CAD build for the part. Positions are in the model's coordinates, mm. Face numbers are marked on the shaded views. A direction names the side the tool comes from. Round coordinates to 2 decimals unless told otherwise and drop trailing zeros. Order: outer loops, then holes, each group sorted by start corner. A loop starts at its lowest first (then second) coordinate and runs counter-clockwise, first axis right, second up. Notation, with made-up numbers: M 65.5,-10 L 82.5,-10 A18 cw 82.5,-5 Z; hole C 52,19.25 d5. An arc over 180 degrees is marked long. Answer as CSV lines item,"result". Start each with the question number.
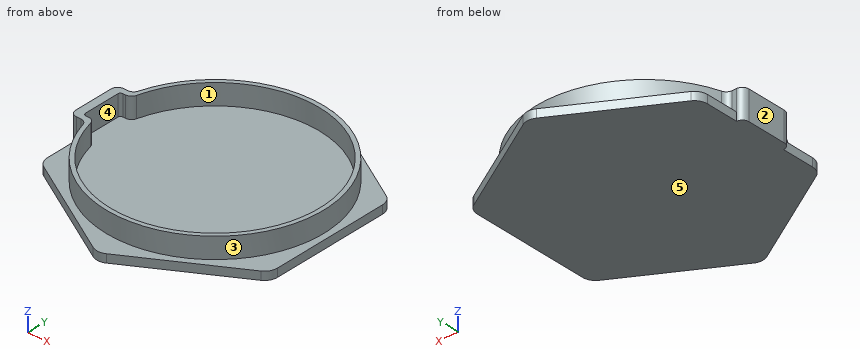
```python
from build123d import *

# Parameters (mm, degrees)
F1_DEPTH = 3.9878
F2_W     = 3.175
F2_H     = 25.4
F3_DEPTH = 3.9878
F5_DEPTH = 9.9822
F6_R     = 6.35
F7_R     = 1.27
F8_R     = 3.175


with BuildPart() as f1:
    # F0 (on Top) → F1 (new body)
    with BuildSketch(Plane.XY):
        Polygon((55.499, 32.042363), (0, 64.084725), (-55.499, 32.042363), (-55.499, -32.042363), (0, -64.084725), (55.499, -32.042363), align=None)
    extrude(amount=F1_DEPTH)

    # F2 (on face) → F3 (join, through all)
    with BuildSketch(Plane.XY.offset(3.9878)):
        with Locations((-57.0865, 0)):
            Rectangle(F2_W, F2_H)
    extrude(amount=-F3_DEPTH)

    # F4 (on face) → F5 (join)
    with BuildSketch(Plane.XY.offset(3.9878)):
        with BuildLine():
            Line((-55.499, -12.7), (-50.955694, -12.7))
            ThreePointArc((-50.955694, -12.7), (52.5145, 0), (-50.955694, 12.7))
            Line((-50.955694, 12.7), (-55.499, 12.7))
            Line((-55.499, 12.7), (-58.674, 12.7))
            Line((-58.674, 12.7), (-58.674, -12.7))
            Line((-58.674, -12.7), (-55.499, -12.7))
        make_face()
        with BuildLine():
            ThreePointArc((-49.483177, 9.9949), (50.4825, 0), (-49.483177, -9.9949))
            Line((-49.483177, -9.9949), (-54.690177, -9.9949))
            Line((-54.690177, -9.9949), (-54.690177, 9.9949))
            Line((-54.690177, 9.9949), (-49.483177, 9.9949))
        make_face(mode=Mode.SUBTRACT)
    extrude(amount=F5_DEPTH)

    # F6
    f6_edges = [f1.edges().sort_by_distance(p)[0] for p in [
        (-55.499, -32.042363, 1.9939),
        (0, -64.084725, 1.9939),
        (55.499, -32.042363, 1.9939),
        (55.499, 32.042363, 1.9939),
        (0, 64.084725, 1.9939),
        (-55.499, 32.042363, 1.9939),
    ]]
    fillet(f6_edges, radius=F6_R)

    # F7
    f7_edges = [f1.edges().sort_by_distance(p)[0] for p in [
        (-54.690177, -9.9949, 8.9789),
        (-54.690177, 9.9949, 8.9789),
    ]]
    fillet(f7_edges, radius=F7_R)

    # F8
    f8_edges = [f1.edges().sort_by_distance(p)[0] for p in [
        (-49.483177, -9.9949, 8.9789),
        (-49.483177, 9.9949, 8.9789),
        (-50.955694, 12.7, 8.9789),
        (-58.674, 12.7, 6.985),
        (-58.674, -12.7, 6.985),
        (-50.955694, -12.7, 8.9789),
    ]]
    fillet(f8_edges, radius=F8_R)


solid = f1.part
```
Q1. Band-saw the part on C-C, the plane y = -47.5. Write the cut outline in (x, z).
Q2. Drop flat-ended pins along their axis: P1, Ø2.5, axis at x = -54.5, z = 7.5, coming from the +Y side; P2, Ø6, axis at x = 31, z = 1.5, coming from the -Y side; P3, Ø2, axis at x = -25.5, y = -31, coming from the +Z side. Give the stop position or say it passes through.
Q3. Mould opens along X. For the marked faces 3, 4 and 5 say: +X half, -X half, draft (parallel to the pull), parting line (faces both ways), or undercut.
Q4. Band-saw the part on B-B, the plane y = 0. Write the cut outline in (x, z).
Q5. Tool access for the marked faces 1 and 2: list every direction of +Z, -Z, +X, -X, +Y, -Y with a clear straight run to the whole face (end or side of a thin tool).
Q6. Band-saw the part on A-A, the plane x = 0. Write the cut outline in (y, z).
Q7. Probe line 1 along X through (y, z) = (0, 8); line 2 along Y through (x, z) = (0, 10.5); line 3 along Z through (x, y) = (-44, 16.5). List the from-to ranges inside material, lowest first. Write a range as from..to.
Answer:
1,outline,"M -28.73,0 L 28.73,0 L 28.73,3.99 L 22.39,3.99 L 22.39,13.97 L 17.09,13.97 L 17.09,3.99 L -17.09,3.99 L -17.09,13.97 L -22.39,13.97 L -22.39,3.99 L -28.73,3.99 Z"
2,P1,"stops at y = 12.7"
2,P2,"stops at y = -47.92"
2,P3,"stops at z = 3.99"
3,face 3,"parting line"
3,face 4,"undercut"
3,face 5,"draft"
4,outline,"M -58.67,0 L 55.5,0 L 55.5,3.99 L 52.51,3.99 L 52.51,13.97 L 50.48,13.97 L 50.48,3.99 L -54.69,3.99 L -54.69,13.97 L -58.67,13.97 Z"
5,face 1,"+Z"
5,face 2,"+Z, -Z, -X, +Y, -Y"
6,outline,"M -63.1,0 L 63.1,0 L 63.1,3.99 L 52.51,3.99 L 52.51,13.97 L 50.48,13.97 L 50.48,3.99 L -50.48,3.99 L -50.48,13.97 L -52.51,13.97 L -52.51,3.99 L -63.1,3.99 Z"
7,line 1,"x = -58.67..-54.69, 50.48..52.51"
7,line 2,"y = -52.51..-50.48, 50.48..52.51"
7,line 3,"z = 0..3.99"
